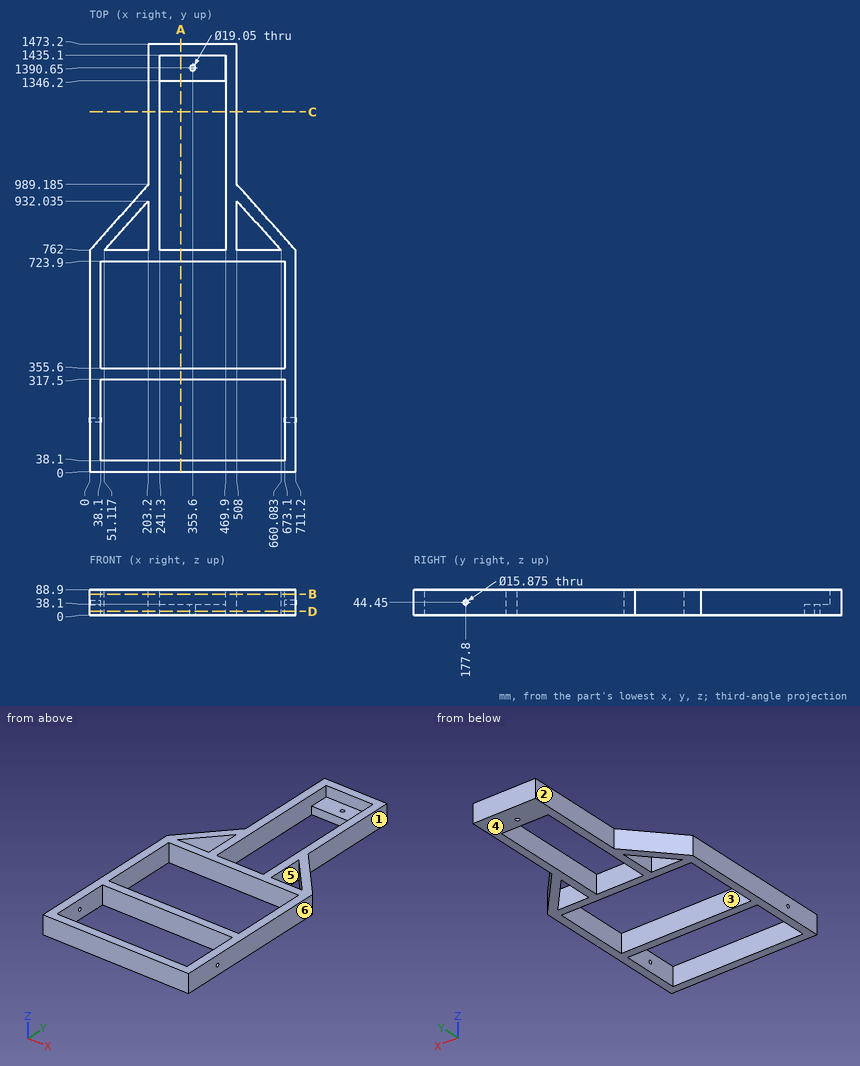
Answer from the drawing. Dimensions are ordinates in mm from the lowest x, y and z of the part. A direction names the side the tool comes from. Coordinates: 2 decimals unless noted, no trailing zeros. Loops run counter-clockwise (first coordinate to the right, second up) from the corner with the lowest first, then second, coordinate; pieces in that order, holes last.
Q1. The part is cut by section C-C on y = 1239. Write down the section's boundary in (x, z), and give its area (3 significant figures).
Q2. Which of the six approach directions +Z, -Z, +X, -X, +Y, -Y give full straight-line access (tool end or side, diameter ignored) to the marked faces 1, 2 and 3?
Q3. Each of these flat-tipped pins is pushed along its axis until it touches: pin 1 Ø2 at (x, z) = (589, 47.5) entering from +Y; pin 2 Ø8 at (y, z) = (973.5, 55) entering from -X (1 decimal); pin 3 Ø19 at (x, z) = (315, 18.5) entering from -Y; pin 4 Ø22 at (x, y) = (355.6, 1390.65) entering from +Z. Where does it stop, or does it pass through?
Q4. The part is cut by section D-D on z = 14. Give the number of separate pieces and of enclosed holes in the cut face, and give its area (3 significant figures).
Q5. Consider probe 1 along Y at (x, z) = (430, 77); probe 2 along Y at (x, z) = (355.6, 9) (1 decimal); probe 3 along X at (y, z) = (1390.65, 9.5) (1 decimal). Determine where each line is inside the solid, lowest interval first.
Q6. The part is cut by section A-A on x = 315. Write down the section's boundary in (y, z).
Q7. The mould has two halves that part along X. Classify the marked faces 4, 5 and 6: +X half, -X half, draft (parallel to the pull), parting line (faces both ways), or undercut.
Q8. The part is cut by section B-B on z = 73.5. Write down the section's boundary in (x, y) (1 decimal), and give its area (3 significant figures).
Results below:
1. outline: (203.2, 0) - (241.3, 0) - (241.3, 88.9) - (203.2, 88.9) - close; (469.9, 0) - (508, 0) - (508, 88.9) - (469.9, 88.9) - close
1. area: 6,770 mm2
2. face 1: +Z, -Z, +X, +Y
2. face 2: +Z, -Z, -X, +Y
2. face 3: +Z, -Z
3. pin 1: stops at y = 899.74
3. pin 2: stops at x = 185.6
3. pin 3: stops at y = 0
3. pin 4: stops at z = 38.1
4. separate pieces: 1
4. enclosed holes: 6
4. area: 234,000 mm2
5. probe 1: y = 0 to 38.1, 317.5 to 355.6, 723.9 to 762, 1435.1 to 1473.2
5. probe 2: y = 0 to 38.1, 317.5 to 355.6, 723.9 to 762, 1346.2 to 1381.1, 1400.2 to 1473.2
5. probe 3: x = 203.2 to 346.1, 365.1 to 508
6. outline: (0, 0) - (38.1, 0) - (38.1, 88.9) - (0, 88.9) - close; (317.5, 0) - (355.6, 0) - (355.6, 88.9) - (317.5, 88.9) - close; (723.9, 0) - (762, 0) - (762, 88.9) - (723.9, 88.9) - close; (1346.2, 0) - (1473.2, 0) - (1473.2, 88.9) - (1435.1, 88.9) - (1435.1, 38.1) - (1346.2, 38.1) - close
7. face 4: draft
7. face 5: undercut
7. face 6: +X half
8. outline: (0, 0) - (711.2, 0) - (711.2, 762) - (508, 989.2) - (508, 1473.2) - (203.2, 1473.2) - (203.2, 989.2) - (0, 762) - close; hole (38.1, 38.1) - (673.1, 38.1) - (673.1, 317.5) - (38.1, 317.5) - close; hole (38.1, 355.6) - (673.1, 355.6) - (673.1, 723.9) - (38.1, 723.9) - close; hole (51.1, 762) - (203.2, 762) - (203.2, 932) - close; hole (241.3, 762) - (469.9, 762) - (469.9, 1435.1) - (241.3, 1435.1) - close; hole (508, 762) - (660.1, 762) - (508, 932) - close
8. area: 214,000 mm2
